```python
from build123d import *

# Parameters (mm, degrees)
SKETCH1_R           = 2
BOSS_EXTRUDE1_DEPTH = 5


with BuildPart() as part:
    # Sketch1 → Boss-Extrude1 (new body)
    with BuildSketch(Plane.XY):
        with BuildLine():
            ThreePointArc((25, 5), (0, 30), (-25, 5))
            Line((-25, 5), (-25, -72.5))
            Line((-25, -72.5), (-10, -72.5))
            Line((-10, -72.5), (-10, -55))
            Line((-10, -55), (10, -55))
            Line((10, -55), (10, -72.5))
            Line((10, -72.5), (25, -72.5))
            Line((25, -72.5), (25, 5))
        make_face()
        Polygon((-10, 20), (-0.75, 20), (-0.75, 27), (0.75, 27), (0.75, 20), (10, 20), (10, -20), (0.75, -20), (0.75, -27), (-0.75, -27), (-0.75, -20), (-10, -20), align=None, mode=Mode.SUBTRACT)
        with Locations((-5, 24)):
            Circle(SKETCH1_R, mode=Mode.SUBTRACT)
        with Locations((5, 24)):
            Circle(SKETCH1_R, mode=Mode.SUBTRACT)
        with Locations((-5, -24)):
            Circle(SKETCH1_R, mode=Mode.SUBTRACT)
        with Locations((5, -24)):
            Circle(SKETCH1_R, mode=Mode.SUBTRACT)
    extrude(amount=BOSS_EXTRUDE1_DEPTH)


solid = part.part
```
Model file for the job. Use its own axes, mm. A direction names the side the tool comes from. Give positions to 0.01 mm unless a question says otherwise; leave off trailing zeros. Write each loop counter-clockwise with the first axis right and the second up, starting at its lowest first coordinate (ties: lowest second). Pieces come first, ordered by that corner, then holes. Notation, with made-up numbers: (-36, 51.25) -> (19, 51.25) arc R17 cw to (19, 69.25) -> close; hole circle Ø5 at (75.25, 20.5). An arc over 180 degrees is marked (long way). Use CSV: the item, a comma, the result in double quotes. Start each with the question number.
1) Two-plate mould, pull along Y, no slides. Class faces 4 (the flat face through (-0.75, -24, 2)), 5 (the flat face through (10, -64, 2)), 6 (the flat face through (17, -72.5, 2)): released by +Y, released by -Y, zero draft, split by the parting line, or undercut.
2) Cut at C-C on x = 5. List the corners of the cut face in (y, z), plus the area to 3 significant figures.
3) Cut at A-A on y = -24. List the corners of the cut face in (x, z).
4) Tool access for faces 1 (the flat face through (-10, -64, 2)), 2 (the flat face through (5, -20, 2)), 3 (the flat face through (25, -34, 2)): list every direction of +Z, -Z, +X, -X, +Y, -Y with a clear straight run to the whole face (end or side of a thin tool).
5) Pin check, flat tips, straight feed: P1, Ø2.5, axis at x = -5, z = 2.5, coming from the -Y side; P2, Ø2, axis at x = 7.5, y = 18.5, coming from the -Z side; P3, Ø2.5, axis at x = 7, z = 2, coming from the +Y side; P4, Ø3, axis at x = 17, z = 1.5, coming from the +Y side. Stop position of each tip, or through.
6) Cut at D-D on y = 0.5. List the corners of the cut face in (x, z).
7) Cut at B-B on z = 0.9. List the corners of the cut face in (x, y), plus the area to 3 significant figures.
8) Drill centre lines: L1, parallel to Y at x = 5, z = 2.05; L2, parallel to X at y = 0, z = 0.55; L3, parallel to X at y = -21, z = 0.9. Where is each one in solid material? Low to high.
Final values:
1,face 4,"undercut"
1,face 5,"zero draft"
1,face 6,"released by -Y"
2,outline,"(-55, 0) -> (-26, 0) -> (-26, 5) -> (-55, 5) -> close; (-22, 0) -> (-20, 0) -> (-20, 5) -> (-22, 5) -> close; (20, 0) -> (22, 0) -> (22, 5) -> (20, 5) -> close; (26, 0) -> (29.49, 0) -> (29.49, 5) -> (26, 5) -> close"
2,area,"182 mm2"
3,outline,"(-25, 0) -> (-7, 0) -> (-7, 5) -> (-25, 5) -> close; (-3, 0) -> (-0.75, 0) -> (-0.75, 5) -> (-3, 5) -> close; (0.75, 0) -> (3, 0) -> (3, 5) -> (0.75, 5) -> close; (7, 0) -> (25, 0) -> (25, 5) -> (7, 5) -> close"
4,face 1,"+Z, -Z, -Y"
4,face 2,"+Z, -Z"
4,face 3,"+Z, -Z, +X, +Y, -Y"
5,P1,"stops at y = -55"
5,P2,"passes through"
5,P3,"stops at y = 29.33"
5,P4,"stops at y = 24.62"
6,outline,"(-25, 0) -> (-10, 0) -> (-10, 5) -> (-25, 5) -> close; (10, 0) -> (25, 0) -> (25, 5) -> (10, 5) -> close"
7,outline,"(-25, -72.5) -> (-10, -72.5) -> (-10, -55) -> (10, -55) -> (10, -72.5) -> (25, -72.5) -> (25, 5) arc R25 ccw to (-25, 5) -> close; hole (-10, -20) -> (-0.75, -20) -> (-0.75, -27) -> (0.75, -27) -> (0.75, -20) -> (10, -20) -> (10, 20) -> (0.75, 20) -> (0.75, 27) -> (-0.75, 27) -> (-0.75, 20) -> (-10, 20) -> close; hole circle Ø4 at (-5, -24); hole circle Ø4 at (-5, 24); hole circle Ø4 at (5, -24); hole circle Ø4 at (5, 24)"
7,area,"3,640 mm2"
8,L1,"y = -55 to -26, -22 to -20, 20 to 22, 26 to 29.49"
8,L2,"x = -25 to -10, 10 to 25"
8,L3,"x = -25 to -0.75, 0.75 to 25"
